Model file for the job. Use its own axes, mm. Face numbers are marked on the shaded views. A direction names the side the tool comes from. Round coordinates to 2 decimals unless told otherwise and drop trailing zeros. Write item = value, one per line.
```python
from build123d import *

# Parameters (mm, degrees)
CROQUIS1_W              = 40.8
CROQUIS1_H              = 40.8
SALIENTE_EXTRUIR1_DEPTH = 11.3
CROQUIS2_W              = 28.1
CROQUIS2_H              = 28.1
SALIENTE_EXTRUIR2_DEPTH = 0.75
REDONDEO1_R             = 1
CROQUIS3_R              = 7.5
SALIENTE_EXTRUIR3_DEPTH = 9
CROQUIS4_R              = 5.8
SALIENTE_EXTRUIR4_DEPTH = 7
CROQUIS5_R              = 11.5
SALIENTE_EXTRUIR5_DEPTH = 2
CROQUIS6_R              = 9.3
SALIENTE_EXTRUIR6_DEPTH = 1.5
REDONDEO4_R             = 10
CROQUIS7_R              = 2.5
SALIENTE_EXTRUIR7_DEPTH = 5
REDONDEO5_R             = 1


with BuildPart() as part:
    # Croquis1 → Saliente-Extruir1 (new, symmetric)
    with BuildSketch(Plane.XY):
        Rectangle(CROQUIS1_W, CROQUIS1_H)
    extrude(amount=SALIENTE_EXTRUIR1_DEPTH, both=True)

    # Croquis2 → Saliente-Extruir2 (add, symmetric)
    with BuildSketch(Plane.XY.offset(11.3)):
        Rectangle(CROQUIS2_W, CROQUIS2_H)
    extrude(amount=SALIENTE_EXTRUIR2_DEPTH, both=True)

    # Redondeo1
    # the kernel refuses this fillet: 1 mm, written as the material it takes off along each edge
    with BuildSketch(Plane(origin=(14.05, 16.470614591, 12.05), x_dir=(0, 0, -1), z_dir=(0, -1, 0)), Plane(origin=(-16.470614591, 14.05, 12.05), x_dir=(0, 0, -1), z_dir=(1, 0, 0)), Plane(origin=(16.470614591, -14.05, 12.05), x_dir=(0, 0, -1), z_dir=(-1, 0, 0)), Plane(origin=(-14.05, -16.470614591, 12.05), x_dir=(0, 0, -1), z_dir=(0, 1, 0))) as redondeo1_piece_1:
        with BuildLine():
            CenterArc((1, -0.968245837), REDONDEO1_R, 104.477512186, 75.522487814)
            Line((0, -0.968245837), (-0.02, -0.968245837))
            Line((-0.02, -0.968245837), (-0.02, 0))
            Line((-0.02, 0), (0, 0.02))
            ThreePointArc((0, 0.02), (0.375, 0.02), (0.745, 0.019364917))
            Line((0.745, 0.019364917), (0.75, 0))
        make_face()
    extrude(amount=32.941229183, mode=Mode.SUBTRACT)

    # Croquis3 → Saliente-Extruir3 (add)
    with BuildSketch(Plane.XY.offset(12.05)):
        Circle(CROQUIS3_R)
    extrude(amount=SALIENTE_EXTRUIR3_DEPTH)

    # Croquis4 → Saliente-Extruir4 (add)
    with BuildSketch(Plane.XY.offset(21.05)):
        Circle(CROQUIS4_R)
    extrude(amount=SALIENTE_EXTRUIR4_DEPTH)

    # Croquis5 → Saliente-Extruir5 (add, symmetric)
    with BuildSketch(Plane.XY.offset(28.05)):
        with Locations((-0.414239482, 0)):
            Circle(CROQUIS5_R)
    extrude(amount=SALIENTE_EXTRUIR5_DEPTH, both=True)

    # Croquis6 → Saliente-Extruir6 (add, symmetric)
    with BuildSketch(Plane.XY.offset(30.05)):
        with Locations((-0.414239482, 0)):
            Circle(CROQUIS6_R)
    extrude(amount=SALIENTE_EXTRUIR6_DEPTH, both=True)

    # Redondeo4
    # the kernel refuses this fillet: 10 mm, written as the material it takes off along each edge
    with BuildSketch(Plane(origin=(-0.414239482, 0, 31.55), x_dir=(1, 0, 0), z_dir=(0, -1, 0))) as redondeo4_piece_1:
        with BuildLine():
            CenterArc((4.032173124, -10), REDONDEO4_R, 58.211669383, 31.788330617)
            Line((4.032173124, 0), (4.032173124, 0.2))
            Line((4.032173124, 0.2), (9.3, 0.2))
            Line((9.3, 0.2), (9.5, 0))
            ThreePointArc((9.5, 0), (9.5, -0.75), (9.405356538, -1.33))
            Line((9.405356538, -1.33), (9.3, -1.5))
        make_face()
    revolve(axis=Axis((-0.414239482, 0, 31.55), (0, 0, 1)), mode=Mode.SUBTRACT)

    # Croquis7 → Saliente-Extruir7 (add)
    with BuildSketch(Plane(origin=(0, 0, -11.3), x_dir=(-1, 0, 0), z_dir=(0, 0, -1))):
        with Locations(Location((-9.4, 11.9, 0), (0, 0, 180))):
            Circle(CROQUIS7_R)
    extrude(amount=SALIENTE_EXTRUIR7_DEPTH)

    # Redondeo5
    redondeo5_edges = [part.edges().sort_by_distance(p)[0] for p in [
        (-20.4, 0, 11.3),
        (0, -20.4, 11.3),
        (20.4, 0, 11.3),
        (0, -20.4, -11.3),
        (-20.4, 0, -11.3),
        (0, 20.4, -11.3),
        (20.4, 0, -11.3),
        (20.4, -20.4, 0),
        (-20.4, -20.4, 0),
        (-20.4, 20.4, 0),
        (20.4, 20.4, 0),
        (0, 20.4, 11.3),
    ]]
    fillet(redondeo5_edges, radius=REDONDEO5_R)


solid = part.part
```
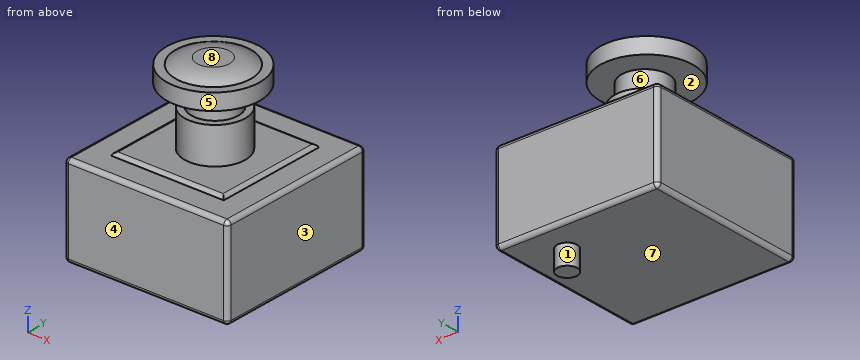
1) 3-axis set-ups, long thin cutter, end or side, ignore diameter. For the marked faces 1, 2, 3, 4 and 5: which of +Z, -Z, +X, -X, +Y, -Y reach the whole face in a straight line?
Conclusion:
face_1 = -Z
face_2 = none
face_3 = +Z, -Z, +X, +Y, -Y
face_4 = +Z, -Z, +X, -X, -Y
face_5 = +Z
2) Wall check: line 1 along Z through (x, y) = (-7.5, -6); line 2 along Z through (x, y) = (7.5, -8); line 3 along Z through (x, y) = (12, -2). Give the ranges that are in metal, low to high.
Conclusion:
line_1 = -11.3 to 12.05, 26.05 to 30.06
line_2 = -11.3 to 12.05, 26.05 to 30.05
line_3 = -11.3 to 12.05
3) Mould opens along Z. For the marked faces 6, 7 and 8 say: +Z half, -Z half, draft (parallel to the pull), parting line (faces both ways), or undercut.
Conclusion:
face_6 = undercut
face_7 = -Z half
face_8 = +Z half
4) Flat gauge pins, fed straight in: pin 1 Ø1.5 at (x, y) = (-9, -7.5) entering from +Z; pin 2 Ø10 at (x, y) = (16, -2.5) entering from +Z; pin 3 Ø10 at (x, y) = (1.5, 2.5) entering from -Z. Where does each tip first touch, or does it go through?
Conclusion:
pin_1 = 30.05
pin_2 = 12.05
pin_3 = -11.3
